from build123d import *

# Parameters (mm, degrees)
SKETCH3_R          = 1.016
CUT_EXTRUDE1_DEPTH = 7.5
CIRPATTERN1_COUNT  = 6


with BuildPart() as part:
    # Sketch1 → Revolve1 (revolve)
    with BuildSketch(Plane(origin=(0, 0, 0), x_dir=(0, 0, -1), z_dir=(1, 0, 0))):
        with BuildLine():
            Line((3.175, 6.5), (12.723311528, 6.5))
            ThreePointArc((12.723311528, 6.5), (14.2875, 0), (12.723311528, -6.5))
            Line((12.723311528, -6.5), (3.175, -6.5))
            Line((3.175, -6.5), (3.175, 6.5))
        make_face()
    revolve(axis=Axis((0, -6.5, 0), (0, 1, 0)))

    # Sketch3 → Cut-Extrude1 (cut, symmetric)
    with BuildSketch(Plane(origin=(0, 0, 0), x_dir=(1, 0, 0), z_dir=(0, 1, 0))):
        with Locations((6.35, 0)):
            Circle(SKETCH3_R)
    cut_extrude1 = extrude(amount=CUT_EXTRUDE1_DEPTH, both=True, mode=Mode.SUBTRACT)

    # CirPattern1: Cut-Extrude1 ×6 about axis
    cirpattern1_axis = Axis((0, 0, 0), (0, 1, 0))
    for i in range(1, CIRPATTERN1_COUNT):
        add(cut_extrude1.rotate(cirpattern1_axis, i * 360 / CIRPATTERN1_COUNT), mode=Mode.SUBTRACT)


solid = part.part
The listing builds one solid part. Answer for the finished solid, in the listing's coordinates (mm). Give positions to 0.01 mm unless a question says otherwise; leave off trailing zeros. Order: outer loops, then holes, each group sorted by start corner. A loop starts at its lowest first (then second) coordinate and runs counter-clockwise, first axis right, second up. Notation, with made-up numbers: (72, 16.25) - (90, 16.25) arc R22 cw to (90, 28.25) - close; hole circle Ø10 at (39, 72.25). An arc over 180 degrees is marked (long way). One line per item, written item: value. Start each with the question number.
1) The mould has two halves that part along Z. Classify faces 1 (the face through (3.92, 0.09, 6.19)), 2 (the face through (3, 6.5, 3)): released by +Z, released by -Z, zero draft, split by the parting line, or undercut.
2) A cutting plane is placed at A-A on x = 0. Give the vertices of the cut face in (y, z) (1 decimal).
3) Given pin 1 Ø1.5 at (x, y) = (-9.5, -4) entering from +Z; pin 2 Ø5 at (x, y) = (-1, -3) entering from -Z; pin 3 Ø2.5 at (x, z) = (3.18, 5.5) entering from +Y; pin 4 Ø1 at (y, z) = (1, 2) entering from +X, each flat-ended and moving along its own axis, determine where each tip first touches the part or whether it passes through.
4) A cutting plane is placed at B-B on z = 0. Give the vertices of the cut face in (x, y) (1 decimal), then the cut area to 3 significant figures.
5) A cutting plane is placed at D-D on y = -0.25. Give the vertices of the cut face in (x, z) (3 decimals), then the cut area to 3 significant figures.
6) Find the intervals of material crossed by L1, parallel to Z at x = -2.75, y = -1.75; L2, parallel to Z at x = 2.25, y = -3.75; L3, parallel to X at y = -0.5, z = 5.5, in increasing order.
7) A cutting plane is placed at C-C on y = 3.75. Give the vertices of the cut face in (x, z) (3 decimals).
Answer sheet:
1. face 1: undercut
1. face 2: zero draft
2. outline: (-6.5, -12.7) arc R14.3 ccw to (6.5, -12.7) - (6.5, -3.2) - (-6.5, -3.2) - close; (-6.5, 3.2) - (6.5, 3.2) - (6.5, 12.7) arc R14.3 ccw to (-6.5, 12.7) - close
3. pin 1: stops at z = 10.62
3. pin 2: stops at z = -14.27
3. pin 3: stops at y = 6.5
3. pin 4: stops at x = 14.18
4. outline: (-12.7, -6.5) - (-7.4, -6.5) - (-7.4, 6.5) - (-12.7, 6.5) arc R14.3 ccw to start; (-5.3, -6.5) - (-3.2, -6.5) - (-3.2, 6.5) - (-5.3, 6.5) - close; (3.2, -6.5) - (5.3, -6.5) - (5.3, 6.5) - (3.2, 6.5) - close; (7.4, -6.5) - (12.7, -6.5) arc R14.3 ccw to (12.7, 6.5) - (7.4, 6.5) - close
4. area: 223 mm2
5. outline: circle Ø28.571 at (0, 0); hole circle Ø2.032 at (-6.35, 0); hole circle Ø2.032 at (-3.175, -5.499); hole circle Ø2.032 at (-3.175, 5.499); hole circle Ø6.35 at (0, 0); hole circle Ø2.032 at (3.175, -5.499); hole circle Ø2.032 at (3.175, 5.499); hole circle Ø2.032 at (6.35, 0)
5. area: 590 mm2
6. L1: z = -13.91 to -6.42, -4.58 to -1.59, 1.59 to 4.58, 6.42 to 13.91
6. L2: z = -13.6 to -5.92, -5.08 to -2.24, 2.24 to 5.08, 5.92 to 13.6
6. L3: x = -13.18 to -4.19, -2.16 to 2.16, 4.19 to 13.18
7. outline: circle Ø27.573 at (0, 0); hole circle Ø2.032 at (-6.35, 0); hole circle Ø2.032 at (-3.175, -5.499); hole circle Ø2.032 at (-3.175, 5.499); hole circle Ø6.35 at (0, 0); hole circle Ø2.032 at (3.175, -5.499); hole circle Ø2.032 at (3.175, 5.499); hole circle Ø2.032 at (6.35, 0)
